Model file for the job. Use its own axes, mm. A direction names the side the tool comes from. Round coordinates to 2 decimals unless told otherwise and drop trailing zeros. Order: outer loops, then holes, each group sorted by start corner. A loop starts at its lowest first (then second) coordinate and runs counter-clockwise, first axis right, second up. Notation, with made-up numbers: (26, 84) -> (47, 84) arc R9 ccw to (47, 89) -> close; hole circle Ø6 at (-21, -29). An arc over 180 degrees is marked (long way). Use CSV: the item, a comma, the result in double quotes.
Autodesk Inventor part; units mm, degrees
ref_plane "YZ Plane" through (0, 0, 0) normal (1, 0, 0) x (0, 1, 0)
ref_plane "XZ Plane" through (0, 0, 0) normal (0, 1, 0) x (-1, 0, 0)
ref_plane "XY Plane" through (0, 0, 0) normal (0, 0, 1) x (1, 0, 0)
sketch "Sketch1" plane through (0, 0, 0) normal (0, 1, 0) x (-1, 0, 0)
  line L0 (40, -25) -> (-40, -25)
  line L1 (-40, -25) -> (-40, 25)
  line L2 (-40, 25) -> (40, 25)
  line L3 (40, 25) -> (40, -25)
  circle A0 centre (30, -5) radius 2.6
  circle A1 centre (0, -7.4) radius 5.59
  circle A2 centre (-30, -5) radius 2.6
  circle A3 centre (10, 15) radius 2.6
  circle A4 centre (-10, 15) radius 2.6
  circle A5 centre (23.57, 16.1) radius 2.5
  circle A6 centre (-23.57, 16.1) radius 2.5
  point P0 (40, 0)
  point P1 (0, 0)
  point P2 (0, -25)
  dimension "d3" = 80
  dimension "d4" = 50
  dimension "d5" = 5.2
  dimension "d6" = 5.2
  dimension "d7" = 5
  dimension "d8" = 11.18
  dimension "d9" = 10
  dimension "d10" = 10
  dimension "d11" = 30
  dimension "d12" = 30
  dimension "d13" = 10
  dimension "d14" = 30
  dimension "d15" = 30
  dimension "d16" = 10
  dimension "d17" = 40
  dimension "d18" = 32.4
  dimension "d19" = 8.9
  dimension "d20" = 8.9
  dimension "d21" = 16.43
  dimension "d44" = 16.43
extrude "Extrusion1" add sketch "Sketch1" along normal blind 12
sketch "Sketch2" plane through (0, 12, 0) normal (0, 1, 0) x (1, 0, 0)
  circle A0 centre (-30, 5) radius 2.6
  circle A1 centre (-10, -15) radius 2.6
  circle A2 centre (10, -15) radius 2.6
  circle A3 centre (30, 5) radius 2.6
  circle A4 centre (-30, 5) radius 4.6
  circle A5 centre (-10, -15) radius 4.6
  circle A6 centre (10, -15) radius 4.6
  circle A7 centre (30, 5) radius 4.6
  point P0 (0, 0)
  dimension "d25" = 9.2
extrude "Extrusion2" cut sketch "Sketch2" against normal blind 1.55 contours A3 | A4 | A5 | A6 | A7
thread "Thread1"
thread "Thread2"
sketch "Sketch3" plane through (0, 0, 0) normal (0, -1, 0) x (1, 0, 0)
  circle A0 centre (0, -7.4) radius 5.59
  circle A1 centre (0, -7.4) radius 8.05
  point P0 (0, 0)
  dimension "d32" = 16.1
extrude "Extrusion3" cut sketch "Sketch3" against normal blind 4.5 contours A0 | A1
sketch "Sketch4" plane through (40, 0, -25) normal (0, 0, -1) x (-1, 0, 0)
  line L0 (0, 0) -> (0, 12)
  point P0 (40, 0)
  point P1 (30, 6)
  point P2 (50, 6)
  point P3 (0, 6)
  dimension "d35" = 30
  dimension "d36" = 20
hole "Hole1" at (10, 6, -25) at (-10, 6, -25) direction (0, 0, 1) diameter 4.134 depth 10
properties part number "C-Beam End Mount" material "Aluminum 6061"
Q1. Cut at A-A (x = -23.57). Give the cut face in (y, z), plus the area to 3 significant figures.
From the geometry:
outline,"(0, -25) -> (12, -25) -> (12, 13.6) -> (0, 13.6) -> close; (0, 18.6) -> (12, 18.6) -> (12, 25) -> (0, 25) -> close"
area,"540 mm²"
Q2. Mould opens along X. For faces 6 (the flat face through (1, 6, 25)), 7 (the cylindrical face through (34.39, 11.24, -6.38)), 8 (the flat face through (-40, 6, 0)) say: +X half, -X half, draft (parallel to the pull), parting line (faces both ways), or undercut.
From the geometry:
face 6,"draft"
face 7,"undercut"
face 8,"-X half"
Q3. Which spindle directions (+Z, -Z, +X, -X, +Y, -Y) get a long thin tool onto all of the face, cutting with end or side? Do faces 1 (the flat face through (10, 6, -15)), 2 (the cylindrical face through (32.6, 5.2, -5.1)), 3 (the flat face through (32, 10.45, -3)), 4 (the flat face through (1, 12, 0)), 5 (the flat face through (2, 4.5, -2)). Say none if no direction does.
From the geometry:
face 1,"-Z"
face 2,"+Y, -Y"
face 3,"+Y"
face 4,"+Z, -Z, +X, -X, +Y"
face 5,"-Y"
Q4. Cut at B-B (y = 6). Give the cut face in (x, z).
From the geometry:
outline,"(-40, -25) -> (-12.07, -25) -> (-12.07, -15) -> (-7.93, -15) -> (-7.93, -25) -> (7.93, -25) -> (7.93, -15) -> (12.07, -15) -> (12.07, -25) -> (40, -25) -> (40, 25) -> (-40, 25) -> close; hole circle Ø5.2 at (-30, -5); hole circle Ø5 at (-23.57, 16.1); hole circle Ø5.2 at (-10, 15); hole circle Ø11.18 at (0, -7.4); hole circle Ø5.2 at (10, 15); hole circle Ø5 at (23.57, 16.1); hole circle Ø5.2 at (30, -5)"
Q5. Cut at D-D (x = 0). Give the cut face in (y, z).
From the geometry:
outline,"(0, -25) -> (12, -25) -> (12, -12.99) -> (4.5, -12.99) -> (4.5, -15.45) -> (0, -15.45) -> close; (0, 0.65) -> (4.5, 0.65) -> (4.5, -1.81) -> (12, -1.81) -> (12, 25) -> (0, 25) -> close"
Q6. Pin check, flat tips, straight feed: pin 1 (3 mm diameter, centred on x = 31, z = -6.5, fed in from +Y); pin 2 (1.2 mm diameter, centred on x = -9.5, y = 5.5, fed in from -Z). Stop position of each tip, or through.
From the geometry:
pin 1,"stops at y = 10.45"
pin 2,"stops at z = -15"
Q7. Probe line 1 along Z through (x, y) = (-30, 3.75); line 2 along X through (y, z) = (2.75, -4); line 3 along X through (y, z) = (9.75, 14.5). List the from-to ranges inside material, lowest first.
From the geometry:
line 1,"z = -25 to -7.6, -2.4 to 25"
line 2,"x = -40 to -32.4, -27.6 to -7.3, 7.3 to 27.6, 32.4 to 40"
line 3,"x = -40 to -25.49, -21.65 to -12.55, -7.45 to 7.45, 12.55 to 21.65, 25.49 to 40"
Q8. Cut at C-C (z = -6). Give the cut face in (x, y).
From the geometry:
outline,"(-40, 0) -> (-32.4, 0) -> (-32.4, 10.45) -> (-34.49, 10.45) -> (-34.49, 12) -> (-40, 12) -> close; (-27.6, 0) -> (-7.93, 0) -> (-7.93, 4.5) -> (-5.41, 4.5) -> (-5.41, 12) -> (-25.51, 12) -> (-25.51, 10.45) -> (-27.6, 10.45) -> close; (5.41, 4.5) -> (7.93, 4.5) -> (7.93, 0) -> (27.6, 0) -> (27.6, 10.45) -> (25.51, 10.45) -> (25.51, 12) -> (5.41, 12) -> close; (32.4, 0) -> (40, 0) -> (40, 12) -> (34.49, 12) -> (34.49, 10.45) -> (32.4, 10.45) -> close"
